```python
from build123d import *

# Parameters (mm, degrees)
SKETCH1_R           = 6.55
BOSS_EXTRUDE4_DEPTH = 5
SKETCH3_W           = 2
SKETCH3_H           = 8.8
SKETCH3_H_2         = 4.1
BOSS_EXTRUDE5_DEPTH = 5
SKETCH4_R           = 6.55
SKETCH4_R_2         = 3
BOSS_EXTRUDE6_DEPTH = 1
CUT_EXTRUDE1_REACH  = 34.342
SKETCH5_R           = 1.5
CUT_EXTRUDE2_REACH  = 34.342
SKETCH6_R           = 1.5


with BuildPart() as part:
    # Sketch1 → Boss-Extrude4 (new body)
    with BuildSketch(Plane(origin=(0, 0, 0), x_dir=(0, 0, -1), z_dir=(1, 0, 0))):
        with BuildLine():
            ThreePointArc((11, 15.35), (8.486364482, 2.35), (11, -10.65))
            Line((11, -10.65), (11, -12.65))
            Line((11, -12.65), (-11, -12.65))
            Line((-11, -12.65), (-11, -10.65))
            ThreePointArc((-11, -10.65), (-8.486364482, 2.35), (-11, 15.35))
            Line((-11, 15.35), (-11, 17.35))
            Line((-11, 17.35), (11, 17.35))
            Line((11, 17.35), (11, 15.35))
        make_face()
        Circle(SKETCH1_R, mode=Mode.SUBTRACT)
        with BuildLine():
            ThreePointArc((8.853997744, -10.65), (7.881360543, -7.696425461), (7.161040408, -4.671402389))
            ThreePointArc((7.161040408, -4.671402389), (0, -8.55), (-7.161040408, -4.671402389))
            ThreePointArc((-7.161040408, -4.671402389), (-7.881360543, -7.696425461), (-8.853997744, -10.65))
            Line((-8.853997744, -10.65), (8.853997744, -10.65))
        make_face(mode=Mode.SUBTRACT)
        with BuildLine():
            Line((-8.853997744, 15.35), (8.853997744, 15.35))
            ThreePointArc((8.853997744, 15.35), (7.389658447, 10.461671711), (6.614219323, 5.41798881))
            ThreePointArc((6.614219323, 5.41798881), (0, 8.55), (-6.614219323, 5.41798881))
            ThreePointArc((-6.614219323, 5.41798881), (-7.389658447, 10.461671711), (-8.853997744, 15.35))
        make_face(mode=Mode.SUBTRACT)
    extrude(amount=BOSS_EXTRUDE4_DEPTH)

    # Sketch3 → Boss-Extrude5 (add)
    with BuildSketch(Plane(origin=(5, 0, 0), x_dir=(0, 0, -1), z_dir=(1, 0, 0))):
        with Locations((0, 10.95)):
            Rectangle(SKETCH3_W, SKETCH3_H)
        with Locations((0, -8.6)):
            Rectangle(SKETCH3_W, SKETCH3_H_2)
    extrude(amount=-BOSS_EXTRUDE5_DEPTH)

    # Sketch4 → Boss-Extrude6 (add)
    with BuildSketch(Plane.ZY):
        Circle(SKETCH4_R)
        Circle(SKETCH4_R_2, mode=Mode.SUBTRACT)
    extrude(amount=-BOSS_EXTRUDE6_DEPTH)

    # Sketch5 → Cut-Extrude1 (cut, up to next)
    with BuildSketch(Plane.XZ.offset(12.65), mode=Mode.PRIVATE) as cut_extrude1_sk1:
        with Locations(Location((2.5, 5, 0), (0, 0, 270))):
            Circle(SKETCH5_R)
    cut_extrude1_tool1 = extrude(cut_extrude1_sk1.sketch, amount=-CUT_EXTRUDE1_REACH, mode=Mode.PRIVATE) & part.part
    # Sketch5 → Cut-Extrude1 (cut, up to next)
    with BuildSketch(Plane.XZ.offset(12.65), mode=Mode.PRIVATE) as cut_extrude1_sk2:
        with Locations(Location((2.5, -5, 0), (0, 0, 90))):
            Circle(SKETCH5_R)
    cut_extrude1_tool2 = extrude(cut_extrude1_sk2.sketch, amount=-CUT_EXTRUDE1_REACH, mode=Mode.PRIVATE) & part.part
    add(cut_extrude1_tool1.solids().sort_by_distance((2.5, -12.65, 5))[0], mode=Mode.SUBTRACT)
    add(cut_extrude1_tool2.solids().sort_by_distance((2.5, -12.65, -5))[0], mode=Mode.SUBTRACT)

    # Sketch6 → Cut-Extrude2 (cut, up to next)
    with BuildSketch(Plane(origin=(0, 17.35, 0), x_dir=(1, 0, 0), z_dir=(0, 1, 0)), mode=Mode.PRIVATE) as cut_extrude2_sk1:
        with Locations(Location((2.5, -5, 0), (0, 0, 90))):
            Circle(SKETCH6_R)
    cut_extrude2_tool1 = extrude(cut_extrude2_sk1.sketch, amount=-CUT_EXTRUDE2_REACH, mode=Mode.PRIVATE) & part.part
    # Sketch6 → Cut-Extrude2 (cut, up to next)
    with BuildSketch(Plane(origin=(0, 17.35, 0), x_dir=(1, 0, 0), z_dir=(0, 1, 0)), mode=Mode.PRIVATE) as cut_extrude2_sk2:
        with Locations(Location((2.5, 5, 0), (0, 0, 270))):
            Circle(SKETCH6_R)
    cut_extrude2_tool2 = extrude(cut_extrude2_sk2.sketch, amount=-CUT_EXTRUDE2_REACH, mode=Mode.PRIVATE) & part.part
    add(cut_extrude2_tool1.solids().sort_by_distance((2.5, 17.35, 5))[0], mode=Mode.SUBTRACT)
    add(cut_extrude2_tool2.solids().sort_by_distance((2.5, 17.35, -5))[0], mode=Mode.SUBTRACT)


solid = part.part
```
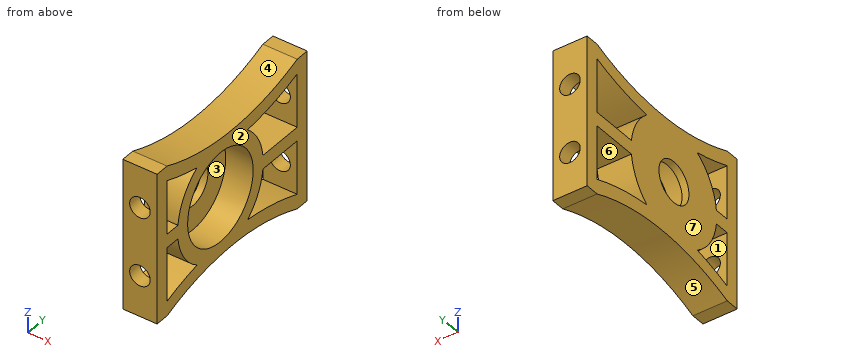
CAD build for the part. Positions are in the model's coordinates, mm. Face numbers are marked on the shaded views. A direction names the side the tool comes from. Give positions to 0.01 mm unless a question says otherwise; leave off trailing zeros. Loops run counter-clockwise (first coordinate to the right, second up) from the corner with the lowest first, then second, coordinate; pieces in that order, holes last. Notation, with made-up numbers: (25.5, 26) -> (67.5, 26) arc R28 cw to (67.5, 53) -> close; hole circle Ø3 at (41.25, -23). An arc over 180 degrees is marked (long way). Use a Markdown table: item, result.
1. Slice it at C-C (z = 4.75). List the corners of the cut face in (x, y).
Check result:
| item | result |
|---|---|
| outline | (0, -12.65) -> (1.02, -12.65) -> (1.02, -10.65) -> (0, -10.65) -> close; (0, -7.11) -> (5, -7.11) -> (5, -4.51) -> (1, -4.51) -> (1, 4.51) -> (5, 4.51) -> (5, 7.11) -> (0, 7.11) -> close; (0, 15.35) -> (1.02, 15.35) -> (1.02, 17.35) -> (0, 17.35) -> close; (3.98, -12.65) -> (5, -12.65) -> (5, -10.65) -> (3.98, -10.65) -> close; (3.98, 15.35) -> (5, 15.35) -> (5, 17.35) -> (3.98, 17.35) -> close |
2. Flat gauge pins, fed straight in: pin 1 (2.5 mm diameter, centred on x = 2, y = 10.5, fed in from +Z); pin 2 (2.5 mm diameter, centred on x = 2.5, z = 5, fed in from +Y); pin 3 (9.5 mm diameter, centred on y = 0, z = 0, fed in from +X). Where does each tip first touch, or does it go through?
Check result:
| item | result |
|---|---|
| pin 1 | stops at z = 9.78 |
| pin 2 | stops at y = 7.68 |
| pin 3 | stops at x = 1 |
3. Slice it at B-B (y = 11). List the corners of the cut face in (x, z).
Check result:
| item | result |
|---|---|
| outline | (0, -9.58) -> (5, -9.58) -> (5, -7.52) -> (0, -7.52) -> close; (0, -1) -> (5, -1) -> (5, 1) -> (0, 1) -> close; (0, 7.52) -> (5, 7.52) -> (5, 9.58) -> (0, 9.58) -> close |
4. Mould opens along Z. For the marked faces 4, 5, 6 and 7 say: pulls with the +Z half, pulls with the -Z half, needs draft (parallel to the pull), parting line crosses it, or undercut.
Check result:
| item | result |
|---|---|
| face 4 | pulls with the +Z half |
| face 5 | pulls with the -Z half |
| face 6 | undercut |
| face 7 | needs draft |
5. Wall check: L1, parallel to Y at x = 0.65, z = 0; L2, parallel to Z at x = 4.6, y = 10.5; L3, parallel to X at y = -11.2, z = 5. Give the ranges that are in metal, low to high. Write a range as [from, to].
Check result:
| item | result |
|---|---|
| L1 | y = [-12.65, -3], [3, 17.35] |
| L2 | z = [-9.45, -7.4], [-1, 1], [7.4, 9.45] |
| L3 | x = [0, 1], [4, 5] |
6. Slice it at A-A (z = 0). List the corners of the cut face in (x, y).
Check result:
| item | result |
|---|---|
| outline | (0, -12.65) -> (5, -12.65) -> (5, -6.55) -> (1, -6.55) -> (1, -3) -> (0, -3) -> close; (0, 3) -> (1, 3) -> (1, 6.55) -> (5, 6.55) -> (5, 17.35) -> (0, 17.35) -> close |
7. Slice it at D-D (y = 0). List the corners of the cut face in (x, z).
Check result:
| item | result |
|---|---|
| outline | (0, -8.57) -> (5, -8.57) -> (5, -6.55) -> (1, -6.55) -> (1, -3) -> (0, -3) -> close; (0, 3) -> (1, 3) -> (1, 6.55) -> (5, 6.55) -> (5, 8.57) -> (0, 8.57) -> close |
8. Which spindle directions (+Z, -Z, +X, -X, +Y, -Y) get a long thin tool onto all of the face, cutting with end or side? Do the marked faces 1, 2 and 3. Say none if no direction does.
Check result:
| item | result |
|---|---|
| face 1 | +X, -X |
| face 2 | +Z, -Z, +X, +Y, -Y |
| face 3 | +X |
